Geometry: see drawing. Coordinates: mm, zero at the bounding-box minimum. Round coordinates to 2 decimals unless told otherwise and drop trailing zeros. Write each loop counter-clockwise with the first axis right and the second up, starting at its lowest first coordinate (ties: lowest second). Pieces come first, ordered by that corner, then holes.
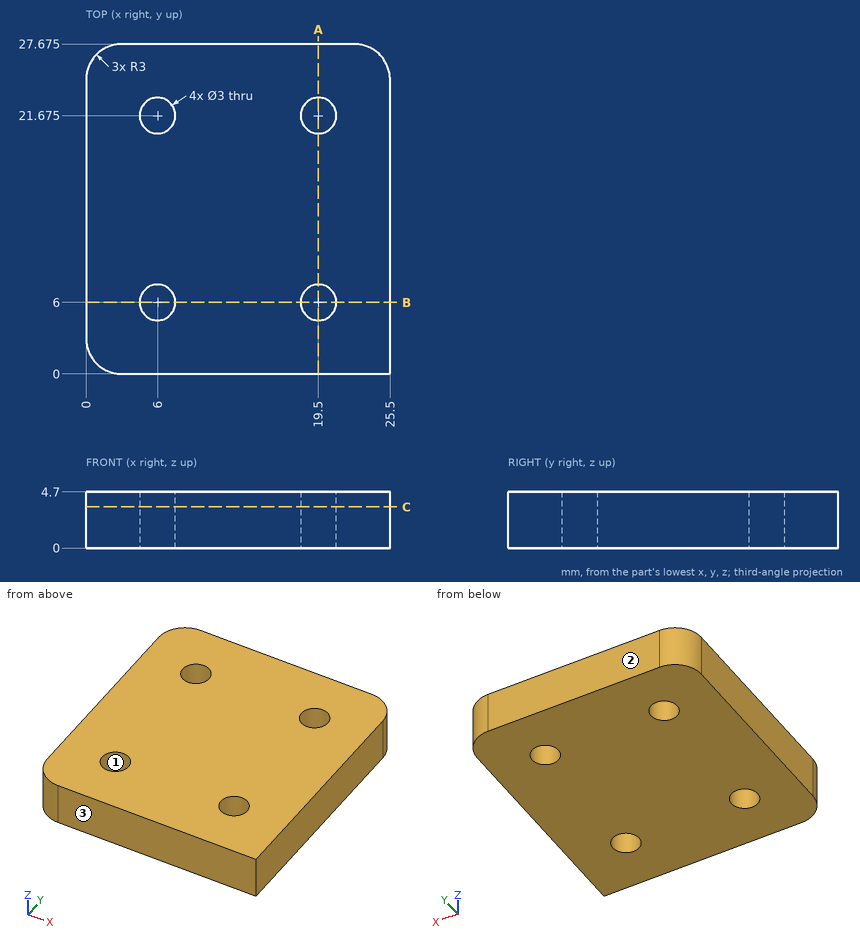
1) Pull-direction query (Y, two-part tool) for the marked faces 1, 2 and 3; classes: released by +Y, released by -Y, zero draft, split by the parting line, or undercut.
Taken from the geometry:
face 1: undercut
face 2: released by +Y
face 3: released by -Y
2) Material intervals for line 1 (Y direction, x = 19.5, z = 3.25) (3 decimals); line 2 (X direction, y = 21.75, z = 1.4); line 3 (X direction, y = 6.5, z = 3.95), sorted ascending.
Taken from the geometry:
line 1: y = 0 to 4.5, 7.5 to 20.175, 23.175 to 27.675
line 2: x = 0 to 4.5, 7.5 to 18, 21 to 25.5
line 3: x = 0 to 4.59, 7.41 to 18.09, 20.91 to 25.5
3) Section query B-B on y = 6. Return the cut outline in (x, z), then the cut area to 4 significant figures.
Taken from the geometry:
outline: (0, 0) - (4.5, 0) - (4.5, 4.7) - (0, 4.7) - close; (7.5, 0) - (18, 0) - (18, 4.7) - (7.5, 4.7) - close; (21, 0) - (25.5, 0) - (25.5, 4.7) - (21, 4.7) - close
area: 91.65 mm2
4) Section query C-C on z = 3.45. Return the cut outline in (x, y) (3 decimals), then the cut area to 3 significant figures.
Taken from the geometry:
outline: (0, 3) arc R3 ccw to (3, 0) - (25.5, 0) - (25.5, 24.675) arc R3 ccw to (22.5, 27.675) - (3, 27.675) arc R3 ccw to (0, 24.675) - close; hole circle Ø3 at (6, 6); hole circle Ø3 at (6, 21.675); hole circle Ø3 at (19.5, 6); hole circle Ø3 at (19.5, 21.675)
area: 672 mm2
5) Section query A-A on x = 19.5. Return the cut outline in (y, z) (3 decimals).
Taken from the geometry:
outline: (0, 0) - (4.5, 0) - (4.5, 4.7) - (0, 4.7) - close; (7.5, 0) - (20.175, 0) - (20.175, 4.7) - (7.5, 4.7) - close; (23.175, 0) - (27.675, 0) - (27.675, 4.7) - (23.175, 4.7) - close
6) Contact query for a flat-ended pin moving along its axis: P1, Ø3, axis at x = 9.5, y = 4, coming from the -Z side. Output: stop coordinate, or through.
Taken from the geometry:
P1: stops at z = 0
